Part print with two shaded views. Sizes in mm from the minimum x, y, z corner. Coordinates: 2 decimals unless noted, no trailing zeros. Order: outer loops, then holes, each group sorted by start corner. A loop starts at its lowest first (then second) coordinate and runs counter-clockwise, first axis right, second up.
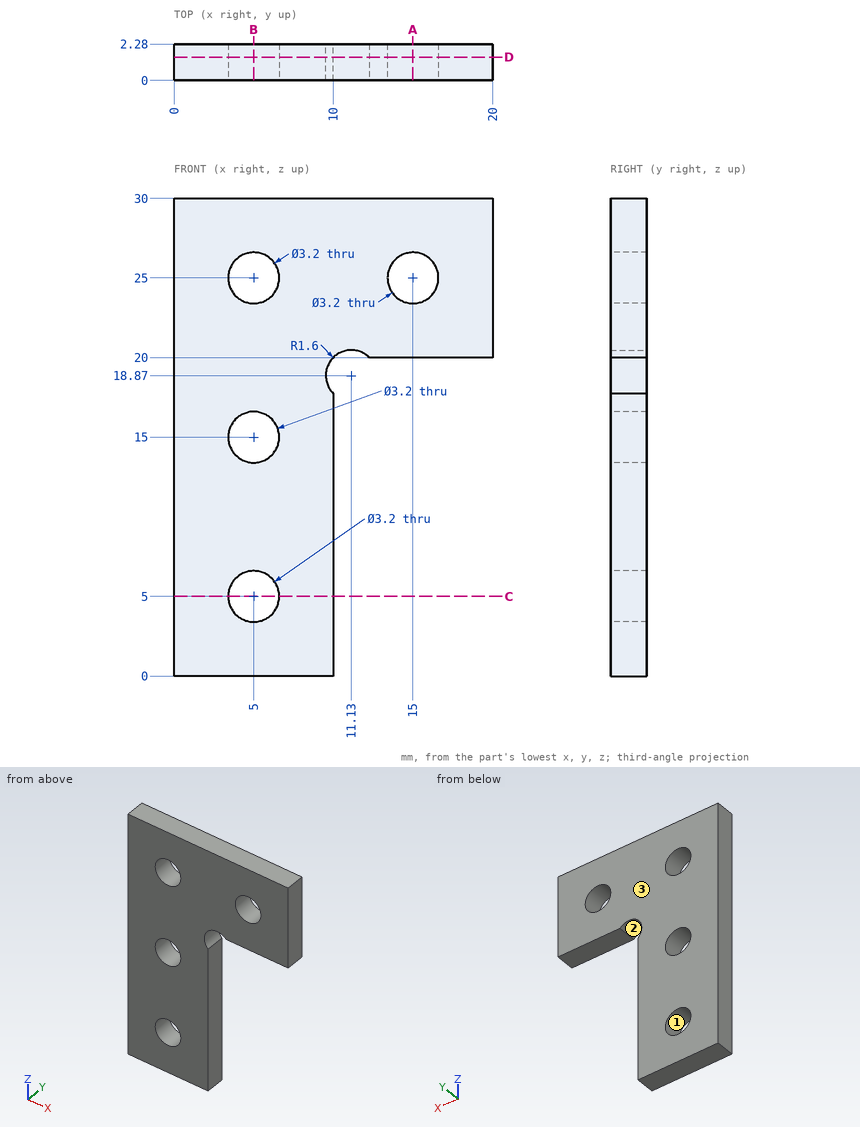
Q1. Cut at D-D on y = 1.45. Write the cut outline in (x, z).
Results list:
outline: (0, 0) - (10, 0) - (10, 17.74) arc R1.6 cw to (12.26, 20) - (20, 20) - (20, 30) - (0, 30) - close; hole circle Ø3.2 at (5, 5); hole circle Ø3.2 at (5, 15); hole circle Ø3.2 at (5, 25); hole circle Ø3.2 at (15, 25)
Q2. Cut at B-B on x = 5. Write the cut outline in (y, z).
Results list:
outline: (0, 0) - (2.28, 0) - (2.28, 3.4) - (0, 3.4) - close; (0, 6.6) - (2.28, 6.6) - (2.28, 13.4) - (0, 13.4) - close; (0, 16.6) - (2.28, 16.6) - (2.28, 23.4) - (0, 23.4) - close; (0, 26.6) - (2.28, 26.6) - (2.28, 30) - (0, 30) - close
Q3. Pin check, flat tips, straight feed: pin 1 Ø1.1 at (y, z) = (1.5, 12) entering from +X; pin 2 Ø0.7 at (x, y) = (14.5, 0.5) entering from -Z. Stop position of each tip, or through.
Results list:
pin 1: stops at x = 10
pin 2: stops at z = 20
Q4. Cut at A-A on x = 15. Write the cut outline in (y, z), and give its area (3 significant figures).
Results list:
outline: (0, 20) - (2.28, 20) - (2.28, 23.4) - (0, 23.4) - close; (0, 26.6) - (2.28, 26.6) - (2.28, 30) - (0, 30) - close
area: 15.5 mm2
Q5. Cut at C-C on z = 5. Write the cut outline in (x, y), and give its area (3 significant figures).
Results list:
outline: (0, 0) - (3.4, 0) - (3.4, 2.28) - (0, 2.28) - close; (6.6, 0) - (10, 0) - (10, 2.28) - (6.6, 2.28) - close
area: 15.5 mm2
Q6. Wall check: line 1 along Z through (x, y) = (5, 1.3); line 2 along Z through (x, y) = (15, 2.1); line 3 along X through (y, z) = (1.75, 25). Give the ranges that are in metal, low to high.
Results list:
line 1: z = 0 to 3.4, 6.6 to 13.4, 16.6 to 23.4, 26.6 to 30
line 2: z = 20 to 23.4, 26.6 to 30
line 3: x = 0 to 3.4, 6.6 to 13.4, 16.6 to 20
Q7. Mould opens along X. For the marked faces 1, 2 and 3 say: pulls with the +X half, pulls with the -X half, needs draft (parallel to the pull), parting line crosses it, or undercut.
Results list:
face 1: undercut
face 2: undercut
face 3: needs draft
